Input: dimensioned drawing with shaded views. Units: mm. Origin: part minimum x, y, z. Round coordinates to 2 decimals unless told otherwise and drop trailing zeros. Loops run counter-clockwise (first coordinate to the right, second up) from the corner with the lowest first, then second, coordinate; pieces in that order, holes last.
1) Section B-B, the plane y = 0.7. Return loops of the section in (x, z) (3 decimals), and give its area (3 significant figures).
2) Ray query, line 1 along Z through (x, y) = (76.36, 0.4) (3 decimals); line 2 along X through (y, z) = (0.9, 45.5); line 3 along X through (y, z) = (1, 9). Return the intervals inside material, ascending.
3) Section C-C, the plane z = 37.5. Return loops of the section in (x, y).
4) Section A-A, the plane x = 27. Return loops of the section in (y, z), and give its area (3 significant figures).
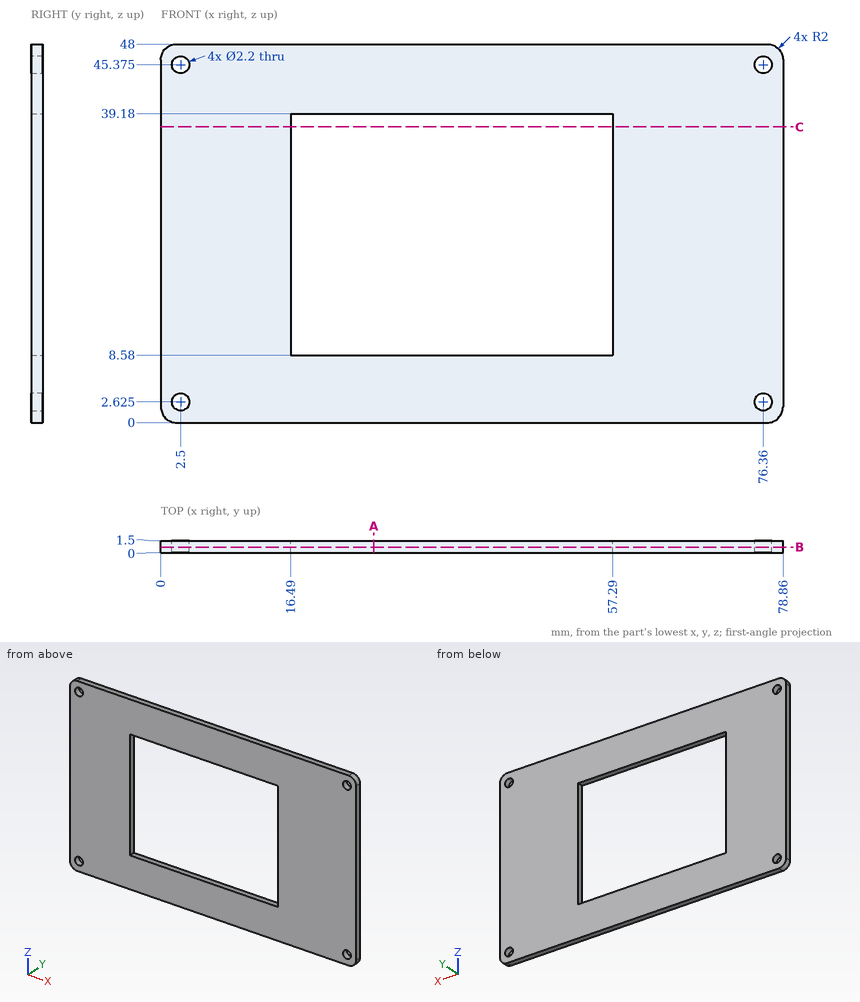
Final values:
1. outline: (0, 2) arc R2 ccw to (2, 0) - (76.86, 0) arc R2 ccw to (78.86, 2) - (78.86, 46) arc R2 ccw to (76.86, 48) - (2, 48) arc R2 ccw to (0, 46) - close; hole circle Ø2.2 at (2.5, 2.625); hole circle Ø2.2 at (2.5, 45.375); hole (16.49, 8.58) - (57.29, 8.58) - (57.29, 39.18) - (16.49, 39.18) - close; hole circle Ø2.2 at (76.36, 2.625); hole circle Ø2.2 at (76.36, 45.375)
1. area: 2,520 mm2
2. line 1: z = 0 to 1.525, 3.725 to 44.275, 46.475 to 48
2. line 2: x = 0 to 1.41, 3.59 to 75.27, 77.45 to 78.86
2. line 3: x = 0 to 16.49, 57.29 to 78.86
3. outline: (0, 0) - (16.49, 0) - (16.49, 1.5) - (0, 1.5) - close; (57.29, 0) - (78.86, 0) - (78.86, 1.5) - (57.29, 1.5) - close
4. outline: (0, 0) - (1.5, 0) - (1.5, 8.58) - (0, 8.58) - close; (0, 39.18) - (1.5, 39.18) - (1.5, 48) - (0, 48) - close
4. area: 26.1 mm2
